```python
from build123d import *

# Parameters (mm, degrees)
F1_ANGLE  = 345
F8_D      = 6
F8_DEPTH  = 12.001
F9_D      = 5
F9_DEPTH  = 12.0010001
F10_D     = 4.5
F10_DEPTH = 12.0010001006
F11_D     = 7
F11_DEPTH = 12.0010001006
F12_D     = 6
F12_DEPTH = 12.001000103
F13_D     = 5
F13_DEPTH = 12.001000103


with BuildPart() as f1:
    # F0 (on Front) → F1 (revolve)
    with BuildSketch(Plane.XZ):
        Polygon((25.1722027957, 100.8808328976), (25.1722027957, 20.8808328976), (28.1722027957, 20.8808328976), (28.1722027957, 14.8808328976), (31.1722027957, 14.8808328976), (31.1722027957, 94.8808328976), (28.1722027957, 94.8808328976), (28.1722027957, 100.8808328976), align=None)
    revolve(axis=Axis((19.1722027957, 0, 37.7046503127), (0, 0, 1)), revolution_arc=F1_ANGLE)

    # F8 (through all, one way)
    with BuildSketch(Plane(origin=(0, 0, 0), x_dir=(1, 0, 0), z_dir=(0, 1, 0))):
        with Locations((19.4538831711, -83.6319848895)):
            Circle(F8_D / 2)
    extrude(amount=-F8_DEPTH, mode=Mode.SUBTRACT)

    # F9 (through all, one way)
    with BuildSketch(Plane(origin=(0, 0, 0), x_dir=(1, 0, 0), z_dir=(0, 1, 0))):
        with Locations((19.1739778966, -68.4388652444)):
            Circle(F9_D / 2)
    extrude(amount=-F9_DEPTH, mode=Mode.SUBTRACT)

    # F10 (through all, one way)
    with BuildSketch(Plane(origin=(0, 0, 0), x_dir=(1, 0, 0), z_dir=(0, 1, 0))):
        with Locations((19.1739778966, -54.2075932026)):
            Circle(F10_D / 2)
    extrude(amount=-F10_DEPTH, mode=Mode.SUBTRACT)

    # F11 (through all, one way)
    with BuildSketch(Plane(origin=(0, 0, 0), x_dir=(1, 0, 0), z_dir=(0, 1, 0))):
        with Locations((19.4538831711, -41.9842377305)):
            Circle(F11_D / 2)
    extrude(amount=-F11_DEPTH, mode=Mode.SUBTRACT)

    # F12 (through all, one way)
    with BuildSketch(Plane(origin=(0, 0, 0), x_dir=(1, 0, 0), z_dir=(0, 1, 0))):
        with Locations((15.0699084625, -28.8323182613)):
            Circle(F12_D / 2)
    extrude(amount=-F12_DEPTH, mode=Mode.SUBTRACT)

    # F13 (through all, one way)
    with BuildSketch(Plane(origin=(0, 0, 0), x_dir=(1, 0, 0), z_dir=(0, 1, 0))):
        with Locations((22.4678628147, -28.8323182613)):
            Circle(F13_D / 2)
    extrude(amount=-F13_DEPTH, mode=Mode.SUBTRACT)


solid = f1.part
```
Geometry: final body of the model. Coordinates: model frame, mm. A direction names the side the tool comes from. Round coordinates to 2 decimals unless told otherwise and drop trailing zeros. Order: outer loops, then holes, each group sorted by start corner. A loop starts at its lowest first (then second) coordinate and runs counter-clockwise, first axis right, second up. Notation, with made-up numbers: (-8.5, 79.25) -> (-2.5, 79.25) arc R30 cw to (-2.5, 101.25) -> close; hole circle Ø6 at (39, 54). An arc over 180 degrees is marked (long way). Use one line per item in the form item = value. Start each with the question number.
1. Draft query along Y for faces 6 (the face through (11.18, 8.95, 55.44)), 7 (the face through (28, 0, 58)), 8 (the face through (24.85, -7.85, 28.08)), 9 (the face through (13, -2, 20.881)). Return one class per face: pulls with the +Y half, pulls with the -Y half, needs draft (parallel to the pull), parting line crosses it, or undercut.
2. Reachability of faces 1 (the face through (27.825, -2.319, 58.483)), 2 (the face through (10.3, 1.5, 17.8)), 3 (the face through (22.225, -8.466, 84.781)), 4 (the face through (13, 0, 100.881)), 5 (the face through (10.3, 1.5, 97.9)) from +Z, -Z, +X, -X, +Y, -Y: full face, straight path, thin tool, end or side. Return the list, or none.
3. Cut plane A-A (y = 7.75). Return the cut outline in (x, z), then the cut area to 3 significant figures.
4. Line query: probe 1 along Y at (x, z) = (18.75, 88.5); probe 2 along Z at (x, y) = (20.5, -10.75); probe 3 along Z at (x, y) = (27, 3.5). Output: solid intervals per line, ascending.
5. Cut plane B-B (z = 59.5). Return the cut outline in (x, y), then the cut area to 3 significant figures.
6. Pin query (flat end, axial travel): pin 1 Ø1.5 at (x, z) = (21, 47.5) entering from -Y; pin 2 Ø1.8 at (x, z) = (29.5, 50.5) entering from -Y; pin 3 Ø12 at (x, y) = (20, -6.5) entering from -Z; pin 4 Ø3.5 at (x, z) = (19.45, 83.63) entering from -Y. Return the tip coordinate at first contact, or that it passes through.
Solution:
q1.face_6 = parting line crosses it
q1.face_7 = undercut
q1.face_8 = needs draft
q1.face_9 = undercut
q2.face_1 = +Z, -Z, +X
q2.face_2 = -Z
q2.face_3 = -Y
q2.face_4 = +Z, +X, -X, +Y, -Y
q2.face_5 = +Z
q3.outline = (10.01, 14.88) -> (14.6, 14.88) -> (14.6, 20.88) -> (23.75, 20.88) -> (23.75, 14.88) -> (28.33, 14.88) -> (28.33, 94.88) -> (23.75, 94.88) -> (23.75, 100.88) -> (14.6, 100.88) -> (14.6, 94.88) -> (10.01, 94.88) -> close
q3.area = 1,470 mm^2
q4.probe_1 = -11.99 to -5.99, 5.99 to 11.99
q4.probe_2 = 14.88 to 27.29, 30.37 to 38.64, 45.32 to 52.39, 56.03 to 66.32, 70.56 to 80.82, 86.44 to 94.88
q4.probe_3 = 20.88 to 100.88
q5.outline = (24.97, -1.55) arc R6 cw (long way) to (25.17, 0) -> (31.17, 0) arc R12 ccw (long way) to (30.76, -3.11) -> close
q5.area = 325 mm^2
q6.pin_1 = -11.95
q6.pin_2 = -7.42
q6.pin_3 = 14.88
q6.pin_4 = 5.65
